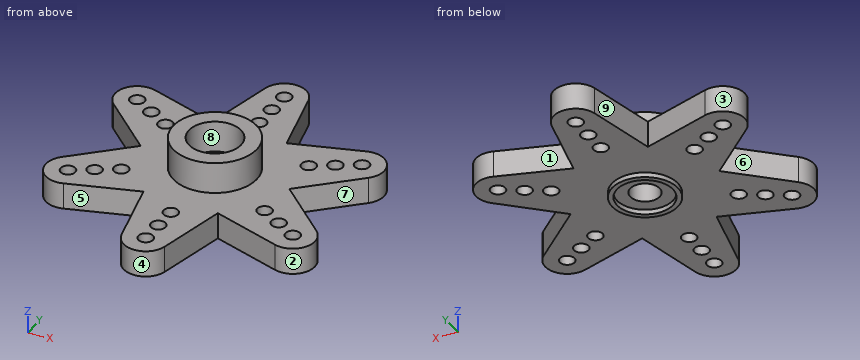
from build123d import *

# Parameters (mm, degrees)
ESBO_O1_R                = 0.75
ESBO_O1_R_2              = 1.5
RESSALTO_EXTRUS_O1_DEPTH = 2.7
PADR_OCIRCULAR1_COUNT    = 6
ESBO_O2_R                = 4.25
ESBO_O2_R_2              = 2.65
RESSALTO_EXTRUS_O2_DEPTH = 3.2
ESBO_O3_R                = 3.35
ESBO_O3_R_2              = 2.85
RESSALTO_EXTRUS_O3_DEPTH = 0.5


with BuildPart() as part:
    # Esboço1 → Ressalto-extrusão1 (new body)
    with BuildSketch(Plane.XY):
        with BuildLine():
            Line((-2.19575939, 13.74106079), (-4.15, 5.002749244))
            ThreePointArc((-4.15, 5.002749244), (0, -6.5), (4.15, 5.002749244))
            Line((4.15, 5.002749244), (2.19575939, 13.74106079))
            ThreePointArc((2.19575939, 13.74106079), (0, 15.5), (-2.19575939, 13.74106079))
        make_face()
        with Locations(Location((0, 13.25, 0), (0, 0, 180))):
            Circle(ESBO_O1_R, mode=Mode.SUBTRACT)
        with Locations(Location((0, 10.85, 0), (0, 0, 180))):
            Circle(ESBO_O1_R, mode=Mode.SUBTRACT)
        with Locations(Location((0, 8.45, 0), (0, 0, 180))):
            Circle(ESBO_O1_R, mode=Mode.SUBTRACT)
        with Locations(Location((0, 0, 0), (0, 0, 180))):
            Circle(ESBO_O1_R_2, mode=Mode.SUBTRACT)
    ressalto_extrus_o1 = extrude(amount=RESSALTO_EXTRUS_O1_DEPTH)

    # PadrãoCircular1: Ressalto-extrusão1 ×6 about axis
    padr_ocircular1_axis = Axis((0, 0, 0), (0, 0, 1))
    for i in range(1, PADR_OCIRCULAR1_COUNT):
        add(ressalto_extrus_o1.rotate(padr_ocircular1_axis, i * 360 / PADR_OCIRCULAR1_COUNT))

    # Esboço2 → Ressalto-extrusão2 (add)
    with BuildSketch(Plane.XY.offset(2.7)):
        Circle(ESBO_O2_R)
        Circle(ESBO_O2_R_2, mode=Mode.SUBTRACT)
    extrude(amount=RESSALTO_EXTRUS_O2_DEPTH)

    # Esboço3 → Ressalto-extrusão3 (add)
    with BuildSketch(Plane(origin=(0, 0, 0), x_dir=(-1, 0, 0), z_dir=(0, 0, -1))):
        with Locations(Location((0, 0, 0), (0, 0, 180))):
            Circle(ESBO_O3_R)
        Circle(ESBO_O3_R_2, mode=Mode.SUBTRACT)
    extrude(amount=RESSALTO_EXTRUS_O3_DEPTH)


solid = part.part
Geometry: final body of the model. Coordinates: model frame, mm. Face numbers are marked on the shaded views. A direction names the side the tool comes from. Give positions to 0.01 mm unless a question says otherwise; leave off trailing zeros. Order: outer loops, then holes, each group sorted by start corner. A loop starts at its lowest first (then second) coordinate and runs counter-clockwise, first axis right, second up. Notation, with made-up numbers: (71, 24.5) -> (110, 24.5) arc R12 ccw to (110, 34.5) -> close; hole circle Ø10 at (65.25, 34). An arc over 180 degrees is marked (long way). Put each result on its own line as item: value.
Q1. Draft query along Y for the marked faces 1, 2, 3 and 4. Return one class per face: released by +Y, released by -Y, zero draft, split by the parting line, or undercut.
Here are the results:
face 1: released by +Y
face 2: undercut
face 3: undercut
face 4: released by -Y
Q2. Section B-B, the plane y = 5.5. Return loops of the section in (x, z).
Here are the results:
outline: (-13.42, 0) -> (-10.14, 0) -> (-10.14, 2.7) -> (-13.42, 2.7) -> close; (-8.65, 0) -> (8.65, 0) -> (8.65, 2.7) -> (-8.65, 2.7) -> close; (10.14, 0) -> (13.42, 0) -> (13.42, 2.7) -> (10.14, 2.7) -> close
Q3. Section A-A, the plane y = 10.85. Return loops of the section in (x, z).
Here are the results:
outline: (-2.84, 0) -> (-0.75, 0) -> (-0.75, 2.7) -> (-2.84, 2.7) -> close; (0.75, 0) -> (2.84, 0) -> (2.84, 2.7) -> (0.75, 2.7) -> close
Q4. Material intervals for L1, parallel to Y at x = -7.25, z = 0.75; L2, parallel to X at y = 10.85, z = 1; L3, parallel to Z at x = -4.25, y = 2.5, sorted ascending.
Here are the results:
L1: y = -7.66 to -4.97, -3.48 to 3.48, 4.97 to 7.66
L2: x = -2.84 to -0.75, 0.75 to 2.84
L3: z = 0 to 2.7
Q5. Section D-D, the plane z = 1.25. Count the separate pieces of the cut face and the enclosed holes in it, then the cut area to 3 significant figures.
Here are the results:
separate pieces: 1
enclosed holes: 19
area: 403 mm^2
Q6. Pin query (flat end, axial travel): pin 1 (2.5 mm diameter, centred on x = -7.32, y = -4.22, fed in from -Z); pin 2 (1.5 mm diameter, centred on x = -7.5, z = 2.5, fed in from +Y); pin 3 (0.9 mm diameter, centred on x = 7.32, y = -4.23, fed in from +Z); pin 4 (2 mm diameter, centred on y = -4, z = 0.5, fed in from +X). Return the tip coordinate at first contact, or that it passes through.
Here are the results:
pin 1: stops at z = 0
pin 2: stops at y = 7.97
pin 3: passes through
pin 4: stops at x = 13.03
Q7. Reachability of the marked faces 5, 6, 7, 8 and 9 from +Z, -Z, +X, -X, +Y, -Y: full face, straight path, thin tool, end or side. Return the list, or none.
Here are the results:
face 5: +Z, -Z, -Y
face 6: +Z, -Z, -X
face 7: +Z, -Z, +X
face 8: +Z
face 9: +Z, -Z, +Y
Q8. Section C-C, the plane z = 4.5. Return loops of the section in (x, y), then the cut area to 3 significant figures.
Here are the results:
outline: circle Ø8.5 at (0, 0); hole circle Ø5.3 at (0, 0)
area: 34.7 mm^2
